CAD build for the part. Positions are in the model's coordinates, mm. Coordinates: 2 decimals unless noted, no trailing zeros. Loops run counter-clockwise (first coordinate to the right, second up) from the corner with the lowest first, then second, coordinate; pieces in that order, holes last. Notation, with made-up numbers: (-1.75, -21.75) -> (52.25, -21.75) arc R20 cw to (52.25, -0.75) -> close; hole circle Ø10 at (85, -10). An arc over 180 degrees is marked (long way). Return JSON: item names as keys, results as strings. Group by question number.
(1) Probe L1, parallel to X at y = 5, z = -118.65; L2, parallel to Z at x = -6.35, y = 1.5; L3, parallel to X at y = 4.75, z = -22. List the from-to ranges inside material, lowest first.
(2) Saw through at A-A on z = -105.95. Write the cut outline in (x, y), then the cut area to 3 significant figures.
(3) Saw through at B-B on y = 1.75. Give the number of separate pieces and of enclosed holes in the cut face, then the cut area to 3 significant figures.
(4) Saw through at C-C on x = -6.35. Write the cut outline in (y, z), then the cut area to 3 significant figures.
(5) Saw through at D-D on x = -56. Write the cut outline in (y, z), then the cut area to 3 significant figures.
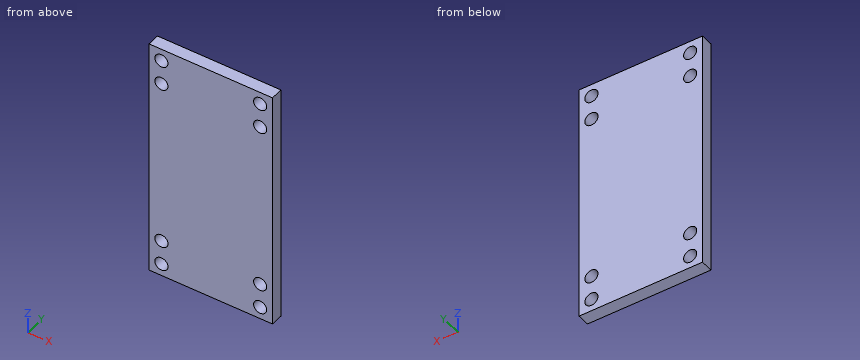
Autodesk Inventor part; units mm, degrees
ref_plane "YZ Plane" through (0, 0, 0) normal (1, 0, 0) x (0, 1, 0)
ref_plane "XZ Plane" through (0, 0, 0) normal (0, 1, 0) x (-1, 0, 0)
ref_plane "XY Plane" through (0, 0, 0) normal (0, 0, 1) x (1, 0, 0)
sketch "Sketch1" plane through (0, 0, 0) normal (0, 1, 0) x (-1, 0, 0)
  line L0 (0, 0) -> (63.5, 0)
  line L1 (63.5, 0) -> (63.5, -125)
  line L2 (63.5, -125) -> (0, -125)
  line L3 (0, -125) -> (0, 0)
  line L4 (63.5, 0) -> (63.5, -6.35)
  line L5 (63.5, -6.35) -> (31.75, -6.35)
  line L6 (31.75, -6.35) -> (57.15, -6.35)
  line L7 (31.75, -6.35) -> (6.35, -6.35)
  line L8 (6.35, -6.35) -> (6.35, -19.05)
  line L9 (57.15, -6.35) -> (57.15, -19.05)
  dimension "d0" = 125
  dimension "d1" = 6.35
  dimension "d2" = 25.4
  dimension "d3" = 63.5
  dimension "d4" = 31.75
  dimension "d5" = 25.4
  dimension "d6" = 12.7
  dimension "d7" = 12.7
extrude "Extrusion1" add sketch "Sketch1" along normal blind 6.35
hole "Hole1" at (-6.35, 0, -6.35) at (-6.35, 0, -19.05) at (-57.15, 0, -6.35) at (-57.15, 0, -19.05) direction (0, 1, 0) diameter 6.7564 end through all
ref_plane "Work Plane1" through (0, 6.35, -62.5) normal (0, 0, 1) x (1, 0, 0)
mirror "Mirror1" about plane through (0, 6.35, -62.5) normal (0, 0, 1) of "Hole1"
properties part number "USAXS Rail Extender"
Geometry results:
{
 "1": {"L1": "-63.5 to -60.53, -53.77 to -9.73, -2.97 to 0", "L2": "-125 to -122.03, -115.27 to -109.33, -102.57 to -22.43, -15.67 to -9.73, -2.97 to 0", "L3": "-63.5 to -58.8, -55.5 to -8, -4.7 to 0"},
 "2": {"outline": "(-63.5, 0) -> (-60.53, 0) -> (-60.53, 6.35) -> (-63.5, 6.35) -> close; (-53.77, 0) -> (-9.73, 0) -> (-9.73, 6.35) -> (-53.77, 6.35) -> close; (-2.97, 0) -> (0, 0) -> (0, 6.35) -> (-2.97, 6.35) -> close", "area": "317 mm²"},
 "3": {"separate pieces": "1", "enclosed holes": "8", "area": "7,650 mm²"},
 "4": {"outline": "(0, -125) -> (6.35, -125) -> (6.35, -122.03) -> (0, -122.03) -> close; (0, -115.27) -> (6.35, -115.27) -> (6.35, -109.33) -> (0, -109.33) -> close; (0, -102.57) -> (6.35, -102.57) -> (6.35, -22.43) -> (0, -22.43) -> close; (0, -15.67) -> (6.35, -15.67) -> (6.35, -9.73) -> (0, -9.73) -> close; (0, -2.97) -> (6.35, -2.97) -> (6.35, 0) -> (0, 0) -> close", "area": "622 mm²"},
 "5": {"outline": "(0, -125) -> (6.35, -125) -> (6.35, -121.83) -> (0, -121.83) -> close; (0, -115.47) -> (6.35, -115.47) -> (6.35, -109.13) -> (0, -109.13) -> close; (0, -102.77) -> (6.35, -102.77) -> (6.35, -22.23) -> (0, -22.23) -> close; (0, -15.87) -> (6.35, -15.87) -> (6.35, -9.53) -> (0, -9.53) -> close; (0, -3.17) -> (6.35, -3.17) -> (6.35, 0) -> (0, 0) -> close", "area": "632 mm²"}
}
